from build123d import *

# Parameters (mm, degrees)
SKETCH029_R     = 1.25
PAD017_DEPTH    = 5.3
SKETCH030_W     = 19.4
SKETCH030_H     = 2.6
PAD018_DEPTH    = 14.3
SKETCH031_R     = 1.25
POCKET009_DEPTH = 2.6


with BuildPart() as part:
    # Sketch029 → Pad017 (new body)
    with BuildSketch(Plane.XY):
        Polygon((-4.5, 0), (4.5, 0), (4.5, -10), (9.7, -10), (9.7, -12.6), (-9.7, -12.6), (-9.7, -10), (-4.5, -10), align=None)
        with Locations((0, -5)):
            Circle(SKETCH029_R, mode=Mode.SUBTRACT)
    extrude(amount=PAD017_DEPTH)

    # Sketch030 (on Face11 of Pad017) → Pad018 (join)
    with BuildSketch(Plane.XY.offset(5.3)):
        with Locations((0, -11.3)):
            Rectangle(SKETCH030_W, SKETCH030_H)
    extrude(amount=PAD018_DEPTH)

    # Sketch031 (on Face7 of Pad018) → Pocket009 (cut)
    with BuildSketch(Plane(origin=(0, -10, 0), x_dir=(-1, 0, 0), z_dir=(0, 1, 0))):
        with Locations((-7.5, 17.45)):
            Circle(SKETCH031_R)
        with Locations((7.5, 17.45)):
            Circle(SKETCH031_R)
    extrude(amount=-POCKET009_DEPTH, mode=Mode.SUBTRACT)


solid = part.part
Model file for the job. Use its own axes, mm. A direction names the side the tool comes from. Give positions to 0.01 mm unless a question says otherwise; leave off trailing zeros. Write each loop counter-clockwise with the first axis right and the second up, starting at its lowest first coordinate (ties: lowest second). Pieces come first, ordered by that corner, then holes. Notation, with made-up numbers: M 0.5,5 L 40.5,5 A18 cw 40.5,12 Z; hole C 85,18 d8. An arc over 180 degrees is marked long. One line per item, written item: value. Start each with the question number.
Q1. Saw through at D-D, the plane x = -6.5. Write the cut outline in (y, z), plus the area to 3 significant figures.
Q2. Saw through at B-B, the plane y = -5. Write the cut outline in (x, z), plus the area to 4 significant figures.
Q3. Probe probe 1 along X at (y, z) = (-10.25, 18.5); probe 2 along Z at (x, y) = (7.5, -11.8); probe 3 along Y at (x, z) = (-4.75, 8.5). List the from-to ranges inside material, lowest first. Write a range as [from, to].
Q4. Saw through at C-C, the plane z = 17.45. Write the cut outline in (x, y), plus the area to 3 significant figures.
Q5. 3-axis set-ups, long thin cutter, end or side, ignore diameter. For faces 4 (the flat face through (0, 0, 3)), 5 (the flat face through (1, -4, 5.3)), 6 (the flat face through (-4.5, -5, 3)): which of +Z, -Z, +X, -X, +Y, -Y reach the whole face in a straight line?
Q6. Drop flat-ended pins along their axis: pin 1 Ø2.5 at (x, y) = (1.5, -4) entering from +Z; pin 2 Ø6 at (y, z) = (-5.5, 2.5) entering from -X; pin 3 Ø2.5 at (y, z) = (-4.5, 2) entering from +X; pin 4 Ø1.5 at (x, y) = (0, -5) entering from -Z. Give the stop position or say it passes through.
Q7. Saw through at A-A, the plane x = 0. Write the cut outline in (y, z), plus the area to 3 significant figures.
Q8. Two-plate mould, pull along X, no slides. Class faces 1 (the flat face through (0, -12.6, 10)), 2 (the cylindrical face through (8.421, -11.282, 18.295)), 3 (the flat face through (4.5, -5, 3)): +X half, -X half, draft (parallel to the pull), parting line (faces both ways), or undercut.
Output values:
1. outline: M -12.6,0 L -10,0 L -10,16.7 L -12.6,16.7 Z; M -12.6,18.2 L -10,18.2 L -10,19.6 L -12.6,19.6 Z
1. area: 47.1 mm²
2. outline: M -4.5,0 L -1.25,0 L -1.25,5.3 L -4.5,5.3 Z; M 1.25,0 L 4.5,0 L 4.5,5.3 L 1.25,5.3 Z
2. area: 34.45 mm²
3. probe 1: x = [-9.7, -8.18], [-6.82, 6.82], [8.18, 9.7]
3. probe 2: z = [0, 16.2], [18.7, 19.6]
3. probe 3: y = [-12.6, -10]
4. outline: M -9.7,-12.6 L -8.75,-12.6 L -8.75,-10 L -9.7,-10 Z; M -6.25,-12.6 L 6.25,-12.6 L 6.25,-10 L -6.25,-10 Z; M 8.75,-12.6 L 9.7,-12.6 L 9.7,-10 L 8.75,-10 Z
4. area: 37.4 mm²
5. face 4: +Z, -Z, +X, -X, +Y
5. face 5: +Z, +X, -X, +Y
5. face 6: +Z, -Z, -X, +Y
6. pin 1: stops at z = 5.3
6. pin 2: stops at x = -4.5
6. pin 3: stops at x = 4.5
6. pin 4: passes through
7. outline: M -12.6,0 L -6.25,0 L -6.25,5.3 L -10,5.3 L -10,19.6 L -12.6,19.6 Z; M -3.75,0 L 0,0 L 0,5.3 L -3.75,5.3 Z
7. area: 90.7 mm²
8. face 1: draft
8. face 2: undercut
8. face 3: +X half
